from build123d import *

# Parameters (mm, degrees)
EXTRUDE_1_DEPTH = 1000


with BuildPart() as part:
    # Эскиз1 → Бобышка-Вытянуть1 (new body)
    with BuildSketch(Plane.XY):
        with BuildLine():
            Line((0, 0), (-6.1, 3.521836642))
            Line((-6.1, 3.521836642), (-5.6, 4.387862046))
            Line((-5.6, 4.387862046), (-5.6, 8.00799361))
            Line((-5.6, 8.00799361), (-6.238589584, 8.00799361))
            ThreePointArc((-6.238589584, 8.00799361), (0, 11), (6.238589584, 8.00799361))
            Line((6.238589584, 8.00799361), (5.6, 8.00799361))
            Line((5.6, 8.00799361), (5.6, 4.387862046))
            Line((5.6, 4.387862046), (6.1, 3.521836642))
            Line((6.1, 3.521836642), (0, 0))
        make_face()
        with BuildLine():
            Line((0, 1.154700538), (-4.6, 3.810511777))
            Line((-4.6, 3.810511777), (-4.6, 8.00799361))
            ThreePointArc((-4.6, 8.00799361), (0, 9.8), (4.6, 8.00799361))
            Line((4.6, 8.00799361), (4.6, 3.810511777))
            Line((4.6, 3.810511777), (0, 1.154700538))
        make_face(mode=Mode.SUBTRACT)
    extrude(amount=EXTRUDE_1_DEPTH)


solid = part.part
Geometry check sheet. Reference: the model listing, model coordinates, mm. Coordinates: 2 decimals unless noted, no trailing zeros. Order: outer loops, then holes, each group sorted by start corner. A loop starts at its lowest first (then second) coordinate and runs counter-clockwise, first axis right, second up. Notation, with made-up numbers: (-32, 80) -> (6, 80) arc R20 cw to (6, 86) -> close; hole circle Ø8 at (-0.75, 15.5). An arc over 180 degrees is marked (long way). Use a Markdown table: item, result. Add a question column.
1. Cross-section at A-A (z = 182). Enter the section's corners in (x, y).
2. Go/stop test with flat-tipped pins: pin 1 Ø4 at (x, z) = (-2, 690) entering from +Y; pin 2 Ø1.5 at (x, z) = (3.5, 597) entering from +Y; pin 3 Ø2 at (y, z) = (9.5, 423.5) entering from +X; pin 4 Ø3.5 at (y, z) = (6, 426.5) entering from +X. Record where each tip stops, or that it passes through.
3. Material ranges on L1, parallel to X at y = 4.5, z = 580.5; L2, parallel to X at y = 4.25, z = 799; L3, parallel to Y at x = 4.5, z = 539.5, recorded low to high.
4. Cross-section at B-B (x = -2.5). Enter the section's corners in (y, z).
Filled sheet:
| question | item | result |
|---|---|---|
| 1 | outline | (-6.24, 8.01) -> (-5.6, 8.01) -> (-5.6, 4.39) -> (-6.1, 3.52) -> (0, 0) -> (6.1, 3.52) -> (5.6, 4.39) -> (5.6, 8.01) -> (6.24, 8.01) arc R8 ccw to start; hole (-4.6, 3.81) -> (0, 1.15) -> (4.6, 3.81) -> (4.6, 8.01) arc R6.8 ccw to (-4.6, 8.01) -> close |
| 2 | pin 1 | y = 11 |
| 2 | pin 2 | y = 10.51 |
| 2 | pin 3 | x = 5.81 |
| 2 | pin 4 | x = 5.68 |
| 3 | L1 | -5.6 to -4.6, 4.6 to 5.6 |
| 3 | L2 | -5.68 to -4.6, 4.6 to 5.68 |
| 3 | L3 | 2.6 to 3.75, 8.1 to 9.61 |
| 4 | outline | (1.44, 0) -> (2.6, 0) -> (2.6, 1000) -> (1.44, 1000) -> close; (9.32, 0) -> (10.6, 0) -> (10.6, 1000) -> (9.32, 1000) -> close |
